The listing builds one solid part. Answer for the finished solid, in the listing's coordinates (mm). Round coordinates to 2 decimals unless told otherwise and drop trailing zeros. Order: outer loops, then holes, each group sorted by start corner. A loop starts at its lowest first (then second) coordinate and runs counter-clockwise, first axis right, second up. Notation, with made-up numbers: (-15, 62.25) - (-4, 62.25) arc R24 ccw to (-4, 81.25) - close; hole circle Ø8 at (50, 25.25). An arc over 180 degrees is marked (long way). Write item = value, one per line.
from build123d import *

# Parameters (mm, degrees)
SKETCH_1_W          = 45
SKETCH_1_H          = 70
SKETCH_1_R          = 1.55
EXTRUDE_1_DEPTH     = 4
SKETCH_3_W          = 70
SKETCH_3_H          = 4
EXTRUDE_3_DEPTH     = 40
SKETCH_4_R          = 2.55
CUT_EXTRUDE_1_DEPTH = 6
CHAMFER_1_SIZE      = 2.5
SKETCH_5_W          = 70
SKETCH_5_H          = 4
EXTRUDE_4_DEPTH     = 10
SKETCH_6_W          = 70
SKETCH_6_H          = 4
EXTRUDE_5_DEPTH     = 10
SKETCH_7_R          = 2.5
CUT_EXTRUDE_2_DEPTH = 10
CHAMFER_3_SIZE      = 2.5


with BuildPart() as part:
    # 草图1 → 凸台-拉伸1 (new body)
    with BuildSketch(Plane(origin=(0, 0, 0), x_dir=(1, 0, 0), z_dir=(0, 1, 0))):
        Rectangle(SKETCH_1_W, SKETCH_1_H)
        with Locations((18.5, 25.5)):
            Circle(SKETCH_1_R, mode=Mode.SUBTRACT)
        with Locations((-18.5, 25.5)):
            Circle(SKETCH_1_R, mode=Mode.SUBTRACT)
        with Locations((-18.5, -25.5)):
            Circle(SKETCH_1_R, mode=Mode.SUBTRACT)
        with Locations((18.5, -25.5)):
            Circle(SKETCH_1_R, mode=Mode.SUBTRACT)
    extrude(amount=EXTRUDE_1_DEPTH)

    # 草图3 → 凸台-拉伸3 (add)
    with BuildSketch(Plane.ZY.offset(22.5)):
        with Locations((0, 2)):
            Rectangle(SKETCH_3_W, SKETCH_3_H)
    extrude(amount=EXTRUDE_3_DEPTH)

    # 草图4 → 切除-拉伸1 (cut)
    with BuildSketch(Plane(origin=(0, 4, 0), x_dir=(1, 0, 0), z_dir=(0, 1, 0))):
        with Locations((-2.5, 0)):
            Circle(SKETCH_4_R)
    extrude(amount=-CUT_EXTRUDE_1_DEPTH, mode=Mode.SUBTRACT)

    # 倒角1
    chamfer_1_edges = [part.edges().sort_by_distance(p)[0] for p in [
        (-5.05, 4, 0),
    ]]
    chamfer(chamfer_1_edges, length=CHAMFER_1_SIZE)

    # 草图5 → 凸台-拉伸4 (add)
    with BuildSketch(Plane(origin=(22.5, 0, 0), x_dir=(0, 0, -1), z_dir=(1, 0, 0))):
        with Locations((0, 2)):
            Rectangle(SKETCH_5_W, SKETCH_5_H)
    extrude(amount=EXTRUDE_4_DEPTH)

    # 草图6 → 凸台-拉伸5 (add)
    with BuildSketch(Plane.ZY.offset(62.5)):
        with Locations((0, 2)):
            Rectangle(SKETCH_6_W, SKETCH_6_H)
    extrude(amount=EXTRUDE_5_DEPTH)

    # 草图7 → 切除-拉伸2 (cut)
    with BuildSketch(Plane(origin=(0, 4, 0), x_dir=(1, 0, 0), z_dir=(0, 1, 0))):
        with Locations((-60.5, 0)):
            Circle(SKETCH_7_R)
    extrude(amount=-CUT_EXTRUDE_2_DEPTH, mode=Mode.SUBTRACT)

    # 倒角3
    chamfer_3_edges = [part.edges().sort_by_distance(p)[0] for p in [
        (-63, 4, 0),
    ]]
    chamfer(chamfer_3_edges, length=CHAMFER_3_SIZE)


solid = part.part
Q1. Section D-D on x = 18.5 is taken. Determine the outline of the cut face in (y, z), then the cut area to 3 significant figures.
Model answer:
outline = (0, -35) - (4, -35) - (4, -27.05) - (0, -27.05) - close; (0, -23.95) - (4, -23.95) - (4, 23.95) - (0, 23.95) - close; (0, 27.05) - (4, 27.05) - (4, 35) - (0, 35) - close
area = 255 mm^2
Q2. Flat-ended cylindrical pins translate along their axes: P1, Ø2, axis at x = 3, z = 8, coming from the -Y side; P2, Ø8, axis at x = -2.5, z = 0, coming from the +Y side; P3, Ø2.5, axis at x = 18.5, z = 25.5, coming from the +Y side (3 decimals). Find the tip coordinate at first contact, or state that the pin passes through.
Model answer:
P1 = 0
P2 = 2.95
P3 = through
Q3. Section B-B on x = -2.5 is taken. Determine the outline of the cut face in (y, z).
Model answer:
outline = (0, -35) - (4, -35) - (4, -5.05) - (1.5, -2.55) - (0, -2.55) - close; (0, 2.55) - (1.5, 2.55) - (4, 5.05) - (4, 35) - (0, 35) - close
Q4. Section A-A on z = 0 is taken. Determine the outline of the cut face in (x, y), then the cut area to 3 significant figures.
Model answer:
outline = (-72.5, 0) - (-63, 0) - (-63, 1.5) - (-65.5, 4) - (-72.5, 4) - close; (-58, 0) - (-5.05, 0) - (-5.05, 1.5) - (-7.55, 4) - (-55.5, 4) - (-58, 1.5) - close; (0.05, 0) - (32.5, 0) - (32.5, 4) - (2.55, 4) - (0.05, 1.5) - close
area = 367 mm^2
Q5. Section C-C on y = 2.65 is taken. Determine the outline of the cut face in (x, z), then the cut area to 3 significant figures.
Model answer:
outline = (-72.5, -35) - (32.5, -35) - (32.5, 35) - (-72.5, 35) - close; hole circle Ø7.3 at (-60.5, 0); hole circle Ø3.1 at (-18.5, -25.5); hole circle Ø3.1 at (-18.5, 25.5); hole circle Ø7.4 at (-2.5, 0); hole circle Ø3.1 at (18.5, -25.5); hole circle Ø3.1 at (18.5, 25.5)
area = 7,230 mm^2
Q6. Find the intervals of material crossed by line 1 (X direction, y = 1, z = 0); line 2 (Z direction, x = -18.5, y = 2.8); line 3 (X direction, y = 2.95, z = -25.5), in increasing order. Write a range as from..to.
Model answer:
line_1 = -72.5..-63, -58..-5.05, 0.05..32.5
line_2 = -35..-27.05, -23.95..23.95, 27.05..35
line_3 = -72.5..-20.05, -16.95..16.95, 20.05..32.5
Q7. Determine the mould class of faces 1 (the face through (-3.079, 1.621, 2.608)), 2 (the face through (-72.5, 2, 0)), 3 (the face through (-19, 2, -35)) for opening direction Z: released by +Z, released by -Z, zero draft, split by the parting line, or undercut.
Model answer:
face_1 = undercut
face_2 = zero draft
face_3 = released by -Z
